```python
from build123d import *

# Parameters (mm, degrees)
SKETCH1_W           = 63
SKETCH1_H           = 30
BOSS_EXTRUDE1_DEPTH = 2
SKETCH2_W           = 63
SKETCH2_H           = 3
BOSS_EXTRUDE2_DEPTH = 12
CUT_EXTRUDE1_DEPTH  = 44.188540147
FILLET1_R           = 3
CUT_EXTRUDE2_DEPTH  = 38.593217473
SKETCH5_R           = 5
CUT_EXTRUDE3_DEPTH  = 1
SKETCH6_R           = 3.25
CUT_EXTRUDE4_DEPTH  = 38.232378382
SKETCH7_R           = 1.5
CUT_EXTRUDE5_DEPTH  = 38.593217473


with BuildPart() as part:
    # Sketch1 → Boss-Extrude1 (new body)
    with BuildSketch(Plane.XY):
        Rectangle(SKETCH1_W, SKETCH1_H)
    extrude(amount=BOSS_EXTRUDE1_DEPTH)

    # Sketch2 → Boss-Extrude2 (add)
    with BuildSketch(Plane.XY):
        with Locations((0, -13.5)):
            Rectangle(SKETCH2_W, SKETCH2_H)
    extrude(amount=-BOSS_EXTRUDE2_DEPTH)

    # Sketch3 → Cut-Extrude1 (cut, through all)
    with BuildSketch(Plane(origin=(0, -12, 0), x_dir=(1, 0, 0), z_dir=(0, 1, 0))):
        with BuildLine():
            Line((25, 6), (25, 18))
            ThreePointArc((25, 18), (26.5, 19.5), (28, 18))
            Line((28, 18), (28, 6))
            ThreePointArc((28, 6), (26.5, 4.5), (25, 6))
        make_face()
        with BuildLine():
            Line((-25, 6), (-25, 18))
            ThreePointArc((-25, 18), (-26.5, 19.5), (-28, 18))
            Line((-28, 18), (-28, 6))
            ThreePointArc((-28, 6), (-26.5, 4.5), (-25, 6))
        make_face()
    extrude(amount=-CUT_EXTRUDE1_DEPTH, mode=Mode.SUBTRACT)

    # Fillet1
    fillet1_edges = [part.edges().sort_by_distance(p)[0] for p in [
        (-31.5, -13.5, -12),
        (31.5, -13.5, -12),
        (-31.5, 15, 1),
        (31.5, 15, 1),
    ]]
    fillet(fillet1_edges, radius=FILLET1_R)

    # Sketch4 → Cut-Extrude2 (cut, through all)
    with BuildSketch(Plane.XY.offset(2)):
        with BuildLine():
            Line((-12, 10.5), (-12, -6.5))
            ThreePointArc((-12, -6.5), (-13.5, -8), (-15, -6.5))
            Line((-15, -6.5), (-15, 10.5))
            ThreePointArc((-15, 10.5), (-13.5, 12), (-12, 10.5))
        make_face()
    extrude(amount=-CUT_EXTRUDE2_DEPTH, mode=Mode.SUBTRACT)

    # Sketch5 → Cut-Extrude3 (cut)
    with BuildSketch(Plane.XY):
        with Locations((-13.5, 2)):
            Circle(SKETCH5_R)
    extrude(amount=CUT_EXTRUDE3_DEPTH, mode=Mode.SUBTRACT)

    # Sketch6 → Cut-Extrude4 (cut, through all)
    with BuildSketch(Plane(origin=(0, 0, 1), x_dir=(-1, 0, 0), z_dir=(0, 0, -1))):
        with Locations((13.5, 2)):
            Circle(SKETCH6_R)
    extrude(amount=-CUT_EXTRUDE4_DEPTH, mode=Mode.SUBTRACT)

    # Sketch7 → Cut-Extrude5 (cut, through all)
    with BuildSketch(Plane.XY.offset(2)):
        with Locations((28.5, 2)):
            Circle(SKETCH7_R)
        with Locations((-1.5, 12)):
            Circle(SKETCH7_R)
        with Locations((-2, -8)):
            Circle(SKETCH7_R)
        with Locations((13, -8)):
            Circle(SKETCH7_R)
    extrude(amount=-CUT_EXTRUDE5_DEPTH, mode=Mode.SUBTRACT)


solid = part.part
```
Build history of the part. All positions in model axes, mm. A direction names the side the tool comes from. Give positions to 0.01 mm unless a question says otherwise; leave off trailing zeros. Order: outer loops, then holes, each group sorted by start corner. A loop starts at its lowest first (then second) coordinate and runs counter-clockwise, first axis right, second up. Notation, with made-up numbers: M -3.75,69 L 37.25,69 A21 ccw 37.25,89 Z; hole C -12.5,81 d5. An arc over 180 degrees is marked long. Return JSON: item names as keys, results as strings.
Q1. 3-axis set-ups, long thin cutter, end or side, ignore diameter. For faces 1 (the face through (-18.5, 2.1, 0.5)), 2 (the face through (-13.5, 12, 1)), 3 (the face through (25, -13, -9)): which of +Z, -Z, +X, -X, +Y, -Y reach the whole face in a straight line?
Answer list:
{"face 1": "-Z", "face 2": "+Z, -Z", "face 3": "-Z, +Y, -Y"}
Q2. Flat gauge pins, fed straight in: pin 1 (4 mm diameter, centred on x = 19.5, z = -5, fed in from +Y); pin 2 (3 mm diameter, centred on x = -16, y = 4, fed in from -Z); pin 3 (0.9 mm diameter, centred on y = -13, z = -10, fed in from -X). Where does each tip first touch, or does it go through?
Answer list:
{"pin 1": "stops at y = -12", "pin 2": "stops at z = 1", "pin 3": "stops at x = -31.45"}
Q3. Two-plate mould, pull along X, no slides. Class faces 4 (the face through (-26.5, -13.5, -4.5)), 5 (the face through (0, 15, 1)), 6 (the face through (30.64, -13.48, -11.1)): pulls with the +X half, pulls with the -X half, needs draft (parallel to the pull), parting line crosses it, or undercut.
Answer list:
{"face 4": "undercut", "face 5": "needs draft", "face 6": "pulls with the +X half"}
Q4. Wall check: probe 1 along X at (y, z) = (-13.5, -9); probe 2 along Y at (x, z) = (13, 1); probe 3 along Z at (x, y) = (-24, 2). Give the ranges that are in metal, low to high. Write a range as from..to.
Answer list:
{"probe 1": "x = -31.5..-28, -25..25, 28..31.5", "probe 2": "y = -15..-9.5, -6.5..15", "probe 3": "z = 0..2"}
Q5. Band-saw the part on B-B (y = -5). Give the cut face in (x, z).
Answer list:
{"outline": "M -31.5,0 L -15,0 L -15,2 L -31.5,2 Z; M -12,0 L 31.5,0 L 31.5,2 L -12,2 Z"}
Q6. Band-saw the part on A-A (x = 13). Give the cut face in (y, z).
Answer list:
{"outline": "M -15,-12 L -12,-12 L -12,0 L -9.5,0 L -9.5,2 L -15,2 Z; M -6.5,0 L 15,0 L 15,2 L -6.5,2 Z"}
Q7. Band-saw the part on D-D (x = 20). Give the cut face in (y, z).
Answer list:
{"outline": "M -15,-12 L -12,-12 L -12,0 L 15,0 L 15,2 L -15,2 Z"}
Q8. Band-saw the part on C-C (x = -1.5). Give the cut face in (y, z), then the cut area to 3 significant figures.
Answer list:
{"outline": "M -15,-12 L -12,-12 L -12,0 L -9.41,0 L -9.41,2 L -15,2 Z; M -6.59,0 L 10.5,0 L 10.5,2 L -6.59,2 Z; M 13.5,0 L 15,0 L 15,2 L 13.5,2 Z", "area": "84.3 mm^2"}
